Part model, mm, in its own coordinate system. Face numbers are marked on the shaded views. Round coordinates to 2 decimals unless told otherwise and drop trailing zeros. Order: outer loops, then holes, each group sorted by start corner. A loop starts at its lowest first (then second) coordinate and runs counter-clockwise, first axis right, second up. Notation, with made-up numbers: (-24.75, 10.5) -> (28.25, 10.5) arc R32 ccw to (28.25, 39.5) -> close; hole circle Ø9 at (8, 66.5). An arc over 180 degrees is marked (long way). Answer as a JSON object with one key per item and string values. Group by question number.
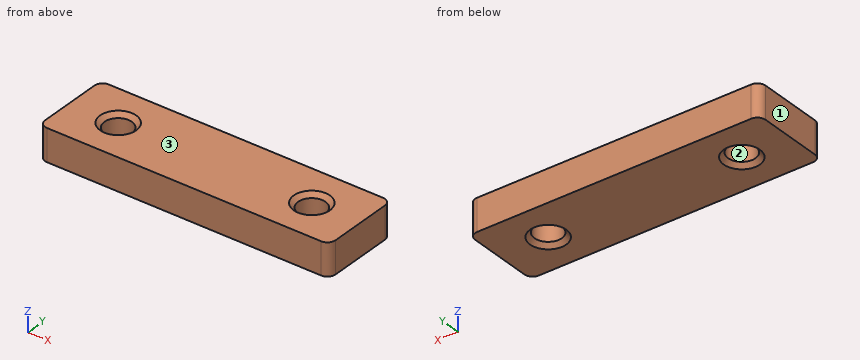
```python
from build123d import *

# Parameters (mm, degrees)
SKETCH1_W                        = 57.15
SKETCH1_H                        = 15.875
BOSS_EXTRUDE1_DEPTH              = 6.35
F_1_4_28_TAPPED_HOLE1_AT_2_COUNT = 2
F_1_4_28_TAPPED_HOLE1_AT_2_PITCH = 38.1
FILLET1_R                        = 1.6002


with BuildPart() as part:
    # Sketch1 → Boss-Extrude1 (new body)
    with BuildSketch(Plane.XY):
        Rectangle(SKETCH1_W, SKETCH1_H)
    extrude(amount=-BOSS_EXTRUDE1_DEPTH)

    # Sketch2 → 1/4-28 Tapped Hole1 (revolve, cut)
    with BuildSketch(Plane(origin=(19.05, 0, 0), x_dir=(0, -1, 0), z_dir=(1, 0, 0))):
        Polygon((0, 0), (0, 6.35), (3.556, 6.35), (2.7051, 5.4991), (2.7051, 0.8509), (3.556, 0), align=None)
    f_1_4_28_tapped_hole1 = revolve(axis=Axis((19.05, 0, 6.35), (0, 0, -1)), mode=Mode.SUBTRACT)

    # 1/4-28 Tapped Hole1 at 2: 1/4-28 Tapped Hole1 ×2
    with Locations(*[(-i * F_1_4_28_TAPPED_HOLE1_AT_2_PITCH, 0, 0) for i in range(1, F_1_4_28_TAPPED_HOLE1_AT_2_COUNT)]):
        add(f_1_4_28_tapped_hole1, mode=Mode.SUBTRACT)

    # Fillet1
    fillet1_edges = [part.edges().sort_by_distance(p)[0] for p in [
        (-28.575, 7.9375, -3.175),
        (28.575, 7.9375, -3.175),
        (28.575, -7.9375, -3.175),
        (-28.575, -7.9375, -3.175),
    ]]
    fillet(fillet1_edges, radius=FILLET1_R)


solid = part.part
```
Q1. Two-plate mould, pull along X, no slides. Class the marked faces 1, 2 and 3: +X half, -X half, draft (parallel to the pull), parting line (faces both ways), or undercut.
Q2. Band-saw the part on B-B (z = -4.25). Count the separate pieces of the cut face and the enclosed holes in it, plus the area to 3 significant figures.
Q3. Wall check: line 1 (X direction, y = 0, z = -4.1) (3 decimals); line 2 (Y direction, x = -19.05, z = -3.35); line 3 (X direction, y = -2, z = -0.5) (3 decimals). Give the ranges that are in metal, low to high. Write a range as [from, to].
Q4. Drop a flat-ended pin along its axis: pin 1 Ø5 at (x, y) = (-19.05, 0) entering from -Z. Give the stop position or say it passes through.
Q5. Band-saw the part on C-C (x = -19.05). List the corners of the cut face in (y, z).
Q6. Band-saw the part on A-A (y = 0). List the corners of the cut face in (x, z) (3 decimals).
Completed:
{
 "1": {"face 1": "-X half", "face 2": "undercut", "face 3": "draft"},
 "2": {"separate pieces": "1", "enclosed holes": "2", "area": "859 mm2"},
 "3": {"line 1": "[-28.575, -21.755], [-16.345, 16.345], [21.755, 28.575]", "line 2": "[-7.94, -2.71], [2.71, 7.94]", "line 3": "[-28.575, -21.361], [-16.739, 16.739], [21.361, 28.575]"},
 "4": {"pin 1": "through"},
 "5": {"outline": "(-7.94, -6.35) -> (-3.56, -6.35) -> (-2.71, -5.5) -> (-2.71, -0.85) -> (-3.56, 0) -> (-7.94, 0) -> close; (2.71, -5.5) -> (3.56, -6.35) -> (7.94, -6.35) -> (7.94, 0) -> (3.56, 0) -> (2.71, -0.85) -> close"},
 "6": {"outline": "(-28.575, -6.35) -> (-22.606, -6.35) -> (-21.755, -5.499) -> (-21.755, -0.851) -> (-22.606, 0) -> (-28.575, 0) -> close; (-16.345, -5.499) -> (-15.494, -6.35) -> (15.494, -6.35) -> (16.345, -5.499) -> (16.345, -0.851) -> (15.494, 0) -> (-15.494, 0) -> (-16.345, -0.851) -> close; (21.755, -5.499) -> (22.606, -6.35) -> (28.575, -6.35) -> (28.575, 0) -> (22.606, 0) -> (21.755, -0.851) -> close"}
}
